```python
from build123d import *

# Parameters (mm, degrees)
BOSS_EXTRUDE1_DEPTH = 5
SKETCH2_R           = 2.5
BOSS_EXTRUDE2_DEPTH = 7.25
SKETCH3_R           = 2.5
BOSS_EXTRUDE3_DEPTH = 7.25


with BuildPart() as part:
    # Sketch1 → Boss-Extrude1 (new, symmetric)
    with BuildSketch(Plane.XY.offset(190)):
        Polygon((-70, 2), (70, 2), (70, 52), (60, 52), (60, 12), (-60, 12), (-60, 52), (-70, 52), align=None)
    extrude(amount=BOSS_EXTRUDE1_DEPTH, both=True)

    # Sketch2 → Boss-Extrude2 (add, symmetric)
    with BuildSketch(Plane(origin=(-77.25, 0, 0), x_dir=(0, 0, -1), z_dir=(1, 0, 0))):
        with Locations(Location((-190, 47, 0), (0, 0, 180))):
            Circle(SKETCH2_R)
    extrude(amount=BOSS_EXTRUDE2_DEPTH, both=True)

    # Sketch3 → Boss-Extrude3 (add, symmetric)
    with BuildSketch(Plane(origin=(77.25, 0, 0), x_dir=(0, 0, -1), z_dir=(1, 0, 0))):
        with Locations(Location((-190, 47, 0), (0, 0, 180))):
            Circle(SKETCH3_R)
    extrude(amount=BOSS_EXTRUDE3_DEPTH, both=True)


solid = part.part
```
Source: CAD feature listing. Evaluate the final solid. Frame: model axes, mm. A direction names the side the tool comes from. Coordinates: 2 decimals unless noted, no trailing zeros. Loops run counter-clockwise (first coordinate to the right, second up) from the corner with the lowest first, then second, coordinate; pieces in that order, holes last. Notation, with made-up numbers: M 68,-30.75 L 106,-30.75 A23 ccw 106,3.25 Z; hole C 59,-7.75 d3. An arc over 180 degrees is marked long. Put each result on its own line as item: value. Start each with the question number.
1) Cut plane D-D on x = 16. Return the cut outline in (y, z).
2) Cut plane A-A on y = 47. Return the cut outline in (x, z), then the cut area to 3 significant figures.
3) Cut plane C-C on y = 17. Return the cut outline in (x, z).
4) Contact query for flat-ended pins moving along their axis: pin 1 Ø2 at (x, z) = (6.5, 189.5) entering from +Y; pin 2 Ø3 at (y, z) = (24.5, 191) entering from -X. Output: stop coordinate, or through.
5) Pull-direction query (X, two-part tool) for faces 4 (the face through (77.35, 47.96, 192.31)), 5 (the face through (-70, 27, 190)), 6 (the face through (-60, 32, 190)), 7 (the face through (1, 12, 190)); classes: pulls with the +X half, pulls with the -X half, needs draft (parallel to the pull), parting line crosses it, or undercut.
6) Reachability of faces 1 (the face through (60, 32, 190)), 2 (the face through (-77.15, 47.96, 192.31)), 3 (the face through (-65, 52, 190)) from +Z, -Z, +X, -X, +Y, -Y: full face, straight path, thin tool, end or side. Return the list, or none.
7) Ray query, L1, parallel to X at y = 12.5, z = 193.5; L2, parallel to Y at x = 18, z = 189; L3, parallel to X at y = 8, z = 189. Return the intervals inside material, ascending. Write a range as from..to.
8) Cut plane B-B on z = 190. Return the cut outline in (x, y).
The answers:
1. outline: M 2,185 L 12,185 L 12,195 L 2,195 Z
2. outline: M -84.5,187.5 L -70,187.5 L -70,185 L -60,185 L -60,195 L -70,195 L -70,192.5 L -84.5,192.5 Z; M 60,185 L 70,185 L 70,187.5 L 84.5,187.5 L 84.5,192.5 L 70,192.5 L 70,195 L 60,195 Z
2. area: 345 mm²
3. outline: M -70,185 L -60,185 L -60,195 L -70,195 Z; M 60,185 L 70,185 L 70,195 L 60,195 Z
4. pin 1: stops at y = 12
4. pin 2: stops at x = -70
5. face 4: needs draft
5. face 5: pulls with the -X half
5. face 6: undercut
5. face 7: undercut
6. face 1: +Z, -Z, +Y
6. face 2: -X
6. face 3: +Z, -Z, +X, -X, +Y
7. L1: x = -70..-60, 60..70
7. L2: y = 2..12
7. L3: x = -70..70
8. outline: M -84.5,44.5 L -70,44.5 L -70,2 L 70,2 L 70,44.5 L 84.5,44.5 L 84.5,49.5 L 70,49.5 L 70,52 L 60,52 L 60,12 L -60,12 L -60,52 L -70,52 L -70,49.5 L -84.5,49.5 Z
